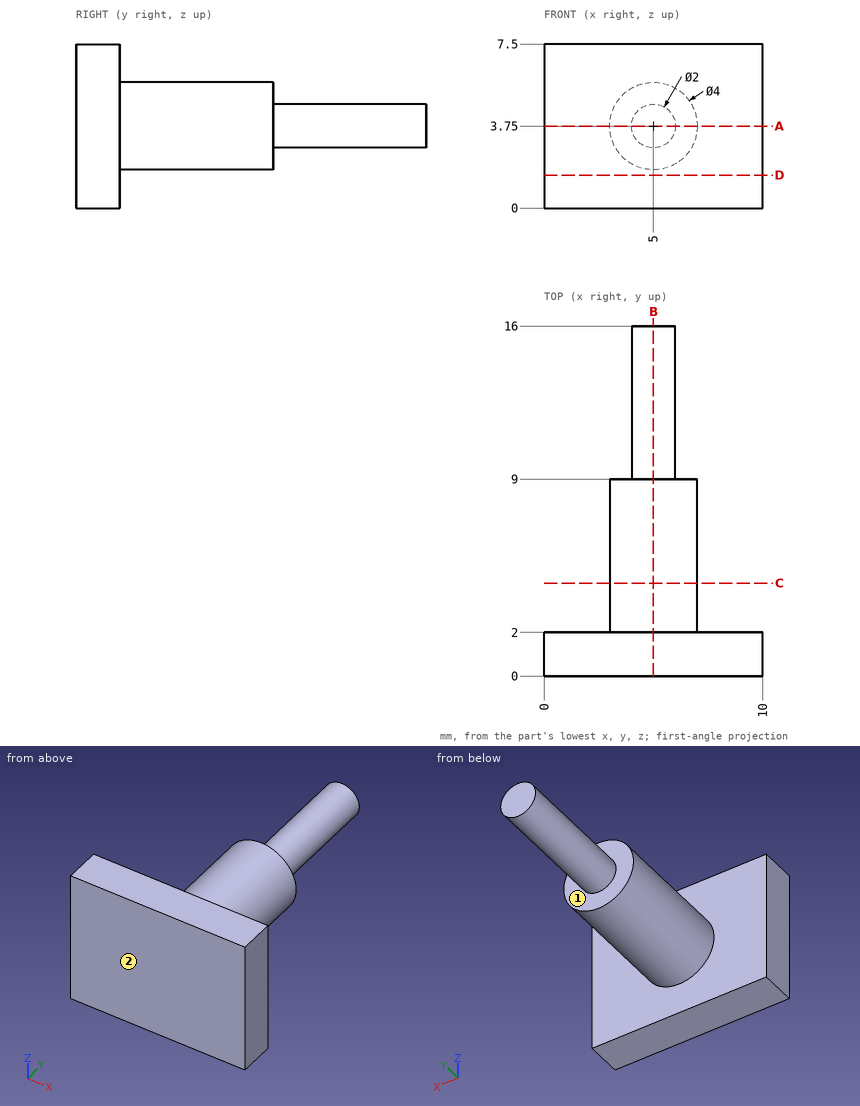
Geometry: see drawing. Coordinates: mm, zero at the bounding-box minimum. A direction names the side the tool comes from. Give positions to 0.01 mm unless a question says otherwise; leave off trailing zeros. Loops run counter-clockwise (first coordinate to the right, second up) from the corner with the lowest first, then second, coordinate; pieces in that order, holes last. Notation, with made-up numbers: M 44.5,19.5 L 79.5,19.5 A19 cw 79.5,55.5 Z; hole C 40.5,-2.75 d1. An arc over 180 degrees is marked long. Answer as CSV lines item,"result". Start each with the question number.
1. Section C-C on y = 4.25. Return loops of the section in (x, z), plus the area to 3 significant figures.
2. Reachability of the marked faces 1 and 2 from +Z, -Z, +X, -X, +Y, -Y: full face, straight path, thin tool, end or side. Return the list, or none.
3. Line query: L1, parallel to Y at x = 6, z = 6; L2, parallel to Y at x = 3.75, z = 5; L3, parallel to X at y = 10, z = 4.25. Output: solid intervals per line, ascending.
4. Pin query (flat end, axial travel): P1, Ø1.5, axis at x = 7.5, y = 5.5, coming from the -Z side; P2, Ø5, axis at x = 6.5, y = 9, coming from the +Z side; P3, Ø1.5, axis at x = 5.5, z = 6.5, coming from the +Y side; P4, Ø2, axis at y = 2, z = 5, coming from the -X side. Return the tip coordinate at first contact, or that it passes through.
5. Section A-A on z = 3.75. Return loops of the section in (x, y).
6. Section D-D on z = 1.5. Return loops of the section in (x, y).
7. Section B-B on x = 5. Return loops of the section in (y, z).
Computed values:
1,outline,"C 5,3.75 d4"
1,area,"12.6 mm²"
2,face 1,"+Y"
2,face 2,"+Z, -Z, +X, -X, -Y"
3,L1,"y = 0 to 2"
3,L2,"y = 0 to 9"
3,L3,"x = 4.13 to 5.87"
4,P1,"stops at z = 2.78"
4,P2,"stops at z = 5.75"
4,P3,"stops at y = 2"
4,P4,"stops at x = 0"
5,outline,"M 0,0 L 10,0 L 10,2 L 7,2 L 7,9 L 6,9 L 6,16 L 4,16 L 4,9 L 3,9 L 3,2 L 0,2 Z"
6,outline,"M 0,0 L 10,0 L 10,2 L 0,2 Z"
7,outline,"M 0,0 L 2,0 L 2,1.75 L 9,1.75 L 9,2.75 L 16,2.75 L 16,4.75 L 9,4.75 L 9,5.75 L 2,5.75 L 2,7.5 L 0,7.5 Z"
